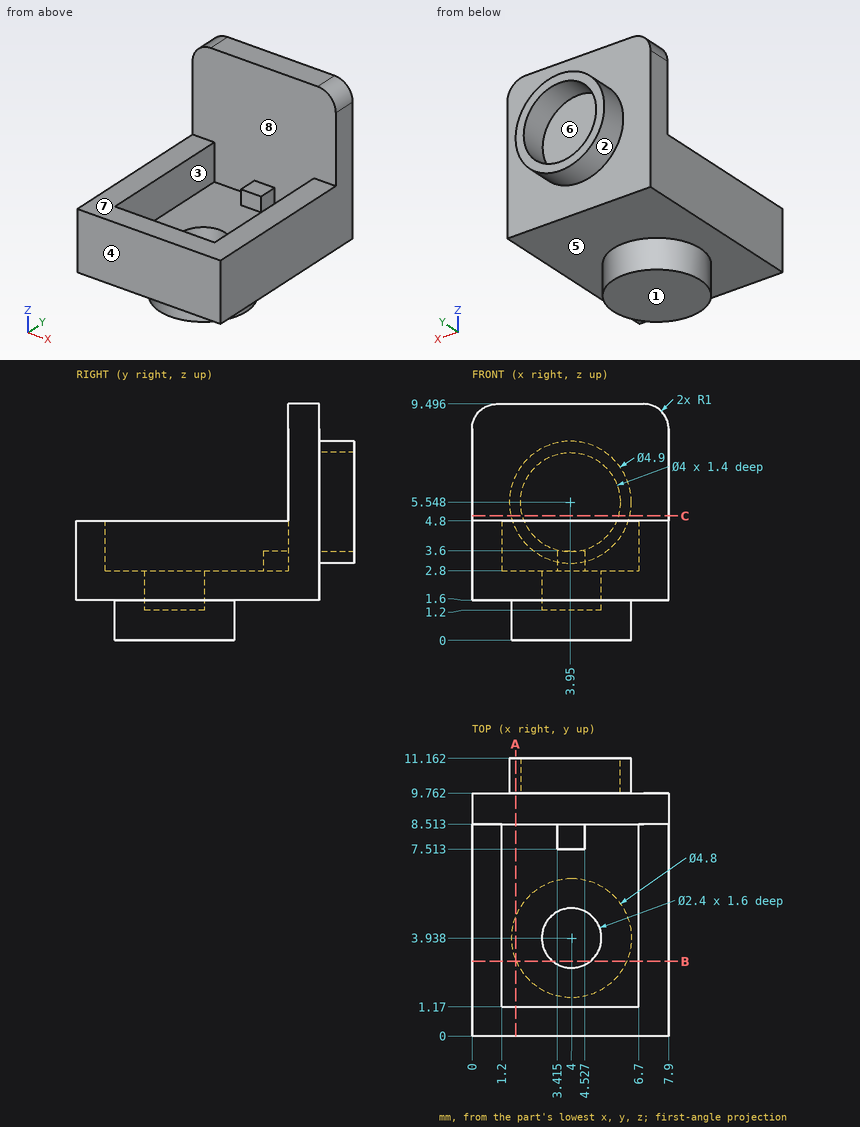
The drawing under review shows one solid part. Ordinate dimensions are in mm from its lowest x, y, z. A direction names the side the tool comes from. Give positions to 0.01 mm unless a question says otherwise; leave off trailing zeros. Write each loop counter-clockwise with the first axis right and the second up, starting at its lowest first coordinate (ties: lowest second). Pieces come first, ordered by that corner, then holes.
1. Draft analysis for pull direction X (two halves, no side actions). For the marked faces 1, 2 and 3, state which applies: +X half, -X half, draft (parallel to the pull), parting line (faces both ways), or undercut.
2. For P1, Ø1.5, axis at x = 2, z = 1.5, coming from the -Y side; P2, Ø0.8, axis at x = 4, y = 8, coming from the +Z side; P3, Ø1, axis at x = 1, z = 7, coming from the +Y side; P4, Ø4.5, axis at x = 4.5, y = 4, coming from the +Z side, all flat-tipped, find the tip position at first contact; note any pin that passes through.
3. Add section B-B, the plane y = 3. Write out the cut boundary in (x, z).
4. Add section C-C, the plane z = 5. Write out the cut boundary in (x, y).
5. Add section A-A, the plane x = 1.75. Write out the cut boundary in (y, z), plus the area to 3 significant figures.
6. Tool access review of the marked faces 4, 5, 6, 7 and 8: name each direction out of +Z, -Z, +X, -X, +Y, -Y from which nothing blocks a thin tool from reaching the whole face with its end or side.
7. Wall thickness on L1, parallel to Y at x = 4, z = 2.4; L2, parallel to Z at x = 3.95, y = 10.1; L3, parallel to Y at x = 1.5, z = 4.75: over which ranges is each line inside the solid? List them lowest first.
Worked answers:
1. face 1: draft
1. face 2: parting line
1. face 3: undercut
2. P1: stops at y = 0
2. P2: stops at z = 3.6
2. P3: stops at y = 9.76
2. P4: stops at z = 4.8
3. outline: (0, 1.6) - (1.79, 1.6) - (1.79, 0) - (6.21, 0) - (6.21, 1.6) - (7.9, 1.6) - (7.9, 4.8) - (6.7, 4.8) - (6.7, 2.8) - (4.75, 2.8) - (4.75, 1.2) - (3.25, 1.2) - (3.25, 2.8) - (1.2, 2.8) - (1.2, 4.8) - (0, 4.8) - close
4. outline: (0, 8.51) - (7.9, 8.51) - (7.9, 9.76) - (6.34, 9.76) - (6.34, 11.16) - (5.87, 11.16) - (5.87, 9.76) - (2.03, 9.76) - (2.03, 11.16) - (1.56, 11.16) - (1.56, 9.76) - (0, 9.76) - close
5. outline: (0, 1.6) - (3.1, 1.6) - (3.1, 0) - (4.77, 0) - (4.77, 1.6) - (9.76, 1.6) - (9.76, 4.47) - (11.16, 4.47) - (11.16, 6.63) - (9.76, 6.63) - (9.76, 9.5) - (8.51, 9.5) - (8.51, 2.8) - (1.17, 2.8) - (1.17, 4.8) - (0, 4.8) - close
5. area: 28.1 mm2
6. face 4: +Z, -Z, +X, -X, -Y
6. face 5: -Z
6. face 6: +Y
6. face 7: +Z, +X, -X, -Y
6. face 8: +Z
7. L1: y = 0 to 2.74, 5.14 to 9.76
7. L2: z = 3.1 to 3.55, 7.55 to 8
7. L3: y = 0 to 1.17, 8.51 to 9.76
